Could you check a few things on this model? Use its own coordinates, in mm. Face numbers are marked on the shaded views. Round coordinates to 2 decimals unless told otherwise and drop trailing zeros. Write each loop counter-clockwise with the first axis right and the second up, starting at its lowest first coordinate (ties: lowest second). Pieces come first, ordered by that corner, then holes. Notation, with made-up numbers: (-28, 86.25) -> (-24, 86.25) arc R4 ccw to (-24, 93.25) -> close; hole circle Ø7 at (52.5, -20.5). An arc over 180 degrees is marked (long way). Answer as CSV lines item,"result". Start each with the question number.
Q1. Imagine slicing it at B-B on y = 15. Please give me the cut outline in (x, z).
Q2. Imagine slicing it at A-A on x = 19.75. Please give me the cut outline in (y, z).
Q3. If I drill on line 1 (Y direction, x = 24.75, z = 4); line 2 (Y direction, x = 20.25, z = 4.5); line 3 (Z direction, x = 26, y = 15), over which ranges is the centre line in solid material (lowest first)? Write a range as [from, to].
Q4. If we mould it in two halves opening along Y, with no side actions, what happens to the marked faces 1, 2, 3 and 4? For each: pulls with the +Y half, pulls with the -Y half, needs draft (parallel to the pull), parting line crosses it, or undercut.
Q5. Imagine slicing it at C-C on x = 27. Please give me the cut outline in (y, z).
Q6. Will these pins go through, and if not, where does the flat tip stop? pin 1 Ø3 at (x, y) = (21, 14.5) entering from +Z; pin 2 Ø4 at (y, z) = (15, 4.5) entering from -X.
Q7. Imagine slicing it at D-D on z = 4.5. Please give me the cut outline in (x, y), and give its area (3 significant figures).
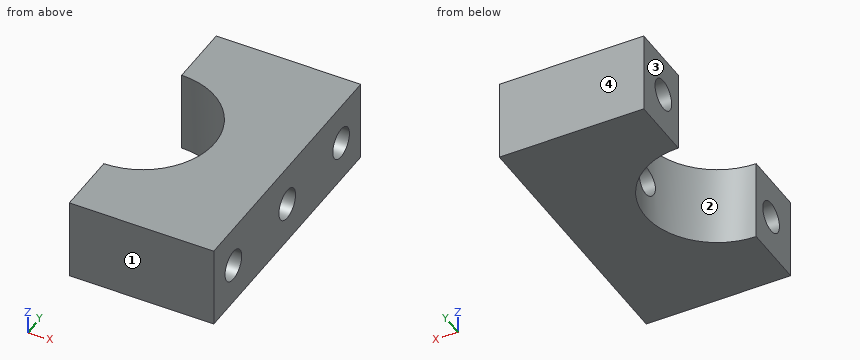
from build123d import *

# Parameters (mm, degrees)
IZIM1_R                     = 7.95
Y_KSEKLIK_EKSTR_ZYON1_DEPTH = 9
IZIM2_R                     = 1.7
KES_EKSTR_ZYON1_DEPTH       = 50
IZIM3_R                     = 1.7
KES_EKSTR_ZYON2_DEPTH       = 29
KES_EKSTR_ZYON3_DEPTH       = 10
Y_KSEKLIK_EKSTR_ZYON2_REACH = 46.777
IZIM5_W                     = 5.408103146
IZIM5_H                     = 14.931073895
IZIM6_R                     = 1.7
KES_EKSTR_ZYON4_DEPTH       = 10


with BuildPart() as part:
    # Çizim1 → Yükseklik-Ekstrüzyon1 (new body)
    with BuildSketch(Plane.XY):
        with BuildLine():
            Line((0, 0), (32, 0))
            Line((32, 0), (32, 8))
            Line((32, 8), (31.5, 8))
            ThreePointArc((31.5, 8), (28.671572875, 9.171572875), (27.5, 12))
            Line((27.5, 12), (27.5, 18))
            ThreePointArc((27.5, 18), (28.671572875, 20.828427125), (31.5, 22))
            Line((31.5, 22), (32, 22))
            Line((32, 22), (32, 30))
            Line((32, 30), (0, 30))
            Line((0, 30), (0, 22))
            Line((0, 22), (0.5, 22))
            ThreePointArc((0.5, 22), (3.328427125, 20.828427125), (4.5, 18))
            Line((4.5, 18), (4.5, 12))
            ThreePointArc((4.5, 12), (3.328427125, 9.171572875), (0.5, 8))
            Line((0.5, 8), (0, 8))
            Line((0, 8), (0, 0))
        make_face()
        with Locations((16, 15)):
            Circle(IZIM1_R, mode=Mode.SUBTRACT)
    extrude(amount=Y_KSEKLIK_EKSTR_ZYON1_DEPTH)

    # Çizim2 → Kes-Ekstrüzyon1 (cut)
    with BuildSketch(Plane(origin=(32, 0, 0), x_dir=(0, 0, -1), z_dir=(1, 0, 0))):
        with Locations((-4.5, 4)):
            Circle(IZIM2_R)
        with Locations((-4.5, 26)):
            Circle(IZIM2_R)
    extrude(amount=-KES_EKSTR_ZYON1_DEPTH, mode=Mode.SUBTRACT)

    # Çizim3 → Kes-Ekstrüzyon2 (cut)
    with BuildSketch(Plane.ZY.offset(-4.5)):
        with Locations(Location((4.5, 15, 0), (0, 0, 270))):
            Circle(IZIM3_R)
    extrude(amount=-KES_EKSTR_ZYON2_DEPTH, mode=Mode.SUBTRACT)

    # Çizim4 → Kes-Ekstrüzyon3 (cut)
    with BuildSketch(Plane(origin=(0, 0, 0), x_dir=(-1, 0, 0), z_dir=(0, 0, -1))):
        Polygon((-16, 30), (-16, 0), (9.241069926, -10.278514345), (11.843794838, 24.557008953), (11.843794838, 39.531622814), align=None)
    extrude(amount=-KES_EKSTR_ZYON3_DEPTH, mode=Mode.SUBTRACT)

    # Yükseklik-Ekstrüzyon2: up to this face of the body (flat: up to its plane)
    y_kseklik_ekstr_zyon2_end = Plane(part.part.faces().sort_by_distance((24.391799767, 15, 9))[0])
    # Çizim5 → Yükseklik-Ekstrüzyon2 (add, up to the picked face)
    with BuildSketch(Plane(origin=(0, 0, 0), x_dir=(-1, 0, 0), z_dir=(0, 0, -1)), mode=Mode.PRIVATE) as y_kseklik_ekstr_zyon2_sk1:
        with Locations((-29.295948427, 14.534463052)):
            Rectangle(IZIM5_W, IZIM5_H)
    y_kseklik_ekstr_zyon2_tool1 = split(extrude(y_kseklik_ekstr_zyon2_sk1.sketch, amount=-Y_KSEKLIK_EKSTR_ZYON2_REACH, mode=Mode.PRIVATE), bisect_by=y_kseklik_ekstr_zyon2_end, keep=Keep.BOTH, mode=Mode.PRIVATE)
    add(y_kseklik_ekstr_zyon2_tool1.solids().sort_by(Axis((29.295948, 14.534463, 0), (0, 0, 1)))[0])

    # Çizim6 → Kes-Ekstrüzyon4 (cut)
    with BuildSketch(Plane.ZY.offset(-26.591896854)):
        with Locations(Location((4.5, 15, 0), (0, 0, 270))):
            Circle(IZIM6_R)
    extrude(amount=-KES_EKSTR_ZYON4_DEPTH, mode=Mode.SUBTRACT)


solid = part.part
Checks:
1,outline,"(23.95, 0) -> (32, 0) -> (32, 2.8) -> (23.95, 2.8) -> close; (23.95, 6.2) -> (32, 6.2) -> (32, 9) -> (23.95, 9) -> close"
2,outline,"(0, 0) -> (7.99, 0) -> (7.99, 9) -> (0, 9) -> close; (22.01, 0) -> (30, 0) -> (30, 9) -> (22.01, 9) -> close; hole circle Ø3.4 at (4, 4.5); hole circle Ø3.4 at (26, 4.5)"
3,line 1,"[0, 2.38], [5.62, 13.38], [16.62, 24.38], [27.62, 30]"
3,line 2,"[0, 2.3], [5.7, 8.28], [21.72, 24.3], [27.7, 30]"
3,line 3,"[0, 2.8], [6.2, 9]"
4,face 1,"pulls with the -Y half"
4,face 2,"undercut"
4,face 3,"needs draft"
4,face 4,"pulls with the +Y half"
5,outline,"(0, 0) -> (30, 0) -> (30, 9) -> (0, 9) -> close; hole circle Ø3.4 at (4, 4.5); hole circle Ø3.4 at (15, 4.5); hole circle Ø3.4 at (26, 4.5)"
6,pin 1,"through"
6,pin 2,"x = 23.69"
7,outline,"(16, 0) -> (32, 0) -> (32, 2.3) -> (16, 2.3) -> close; (16, 5.7) -> (32, 5.7) -> (32, 13.3) -> (23.77, 13.3) arc R7.95 cw to (16, 7.05) -> close; (16, 22.95) arc R7.95 cw to (23.77, 16.7) -> (32, 16.7) -> (32, 24.3) -> (16, 24.3) -> close; (16, 27.7) -> (32, 27.7) -> (32, 30) -> (16, 30) -> close"
7,area,"244 mm^2"
